```python
from build123d import *

# Parameters (mm, degrees)
F0_W     = 190
F0_H     = 130
F1_DEPTH = 8
F2_R     = 25
F3_R     = 3


with BuildPart() as f1:
    # F0 (on Top) → F1 (new body)
    with BuildSketch(Plane.XY):
        Rectangle(F0_W, F0_H)
    extrude(amount=F1_DEPTH)

    # F2
    f2_edges = [f1.edges().sort_by_distance(p)[0] for p in [
        (-95, 65, 4),
        (-95, -65, 4),
        (95, -65, 4),
        (95, 65, 4),
    ]]
    fillet(f2_edges, radius=F2_R)

    # F3
    f3_edges = [f1.edges().sort_by_distance(p)[0] for p in [
        (0, 65, 8),
        (87.67767, 57.67767, 8),
        (-87.67767, 57.67767, 8),
        (95, 0, 8),
        (-95, 0, 8),
        (87.67767, -57.67767, 8),
        (-87.67767, -57.67767, 8),
        (0, -65, 8),
    ]]
    fillet(f3_edges, radius=F3_R)


solid = f1.part
```
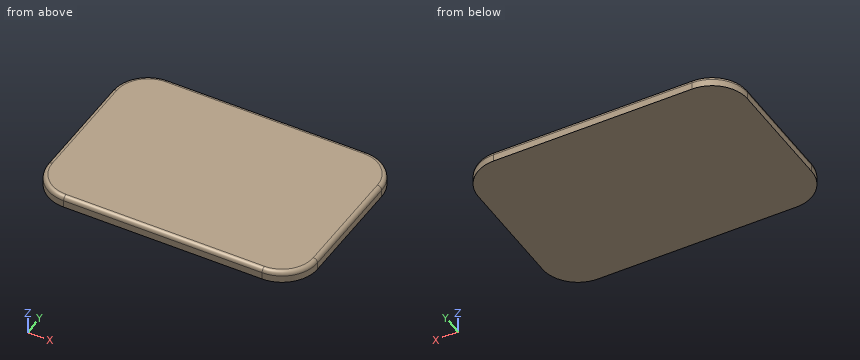
Geometry: final body of the model. Coordinates: model frame, mm. Give positions to 0.01 mm unless a question says otherwise; leave off trailing zeros. Loops run counter-clockwise (first coordinate to the right, second up) from the corner with the lowest first, then second, coordinate; pieces in that order, holes last. Notation, with made-up numbers: (19.5, -32) -> (53.5, -32) arc R26 cw to (53.5, -13) -> close; hole circle Ø8 at (8.25, 17). An arc over 180 degrees is marked (long way). Use one line per item in the form item = value.
Item 1: Pin query (flat end, axial travel): P1, Ø3, axis at y = 42.5, z = 1.5, coming from the +X side. Return the tip coordinate at first contact, or that it passes through.
A:
P1 = 94.98
Item 2: Section query A-A on z = 3.5. Output: boundary loops of the cut face in (x, y), and give its area (3 significant figures).
A:
outline = (-95, -40) arc R25 ccw to (-70, -65) -> (70, -65) arc R25 ccw to (95, -40) -> (95, 40) arc R25 ccw to (70, 65) -> (-70, 65) arc R25 ccw to (-95, 40) -> close
area = 24,200 mm^2
Item 3: Line query: probe 1 along X at (y, z) = (-58, 6.75); probe 2 along Y at (x, z) = (-75.5, 2.5); probe 3 along X at (y, z) = (57.5, 3.75). Output: solid intervals per line, ascending.
A:
probe_1 = -86.53 to 86.53
probe_2 = -64.39 to 64.39
probe_3 = -87.85 to 87.85
